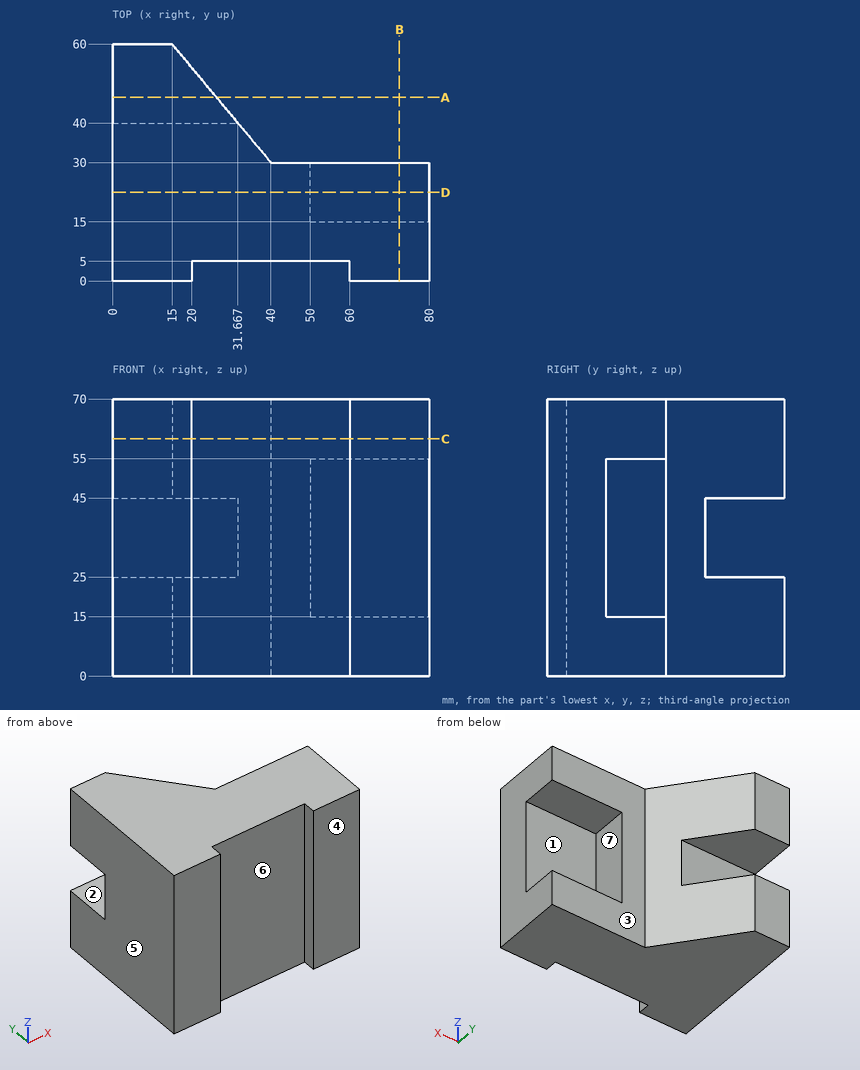
The drawing under review shows one solid part. Ordinate dimensions are in mm from its lowest x, y, z. A direction names the side the tool comes from. Give positions to 0.01 mm unless a question says otherwise; leave off trailing zeros. Loops run counter-clockwise (first coordinate to the right, second up) from the corner with the lowest first, then second, coordinate; pieces in that order, holes last. Notation, with made-up numbers: M 54,86 L 80,86 A22 ccw 80,108 Z; hole C 46,-32 d8. An arc over 180 degrees is marked long. One line per item, written item: value. Start each with the question number.
Q1. Add section C-C (z = 60). Give the boundary of the cut face in (x, y).
Q2. Draft analysis for pull direction X (two halves, no side actions). For the marked faces 4, 5, 6 and 7, state which applies: released by +X, released by -X, zero draft, split by the parting line, or undercut.
Q3. Machinability: for the marked faces 1, 2 and 3, which of the approach directions +Z, -Z, +X, -X, +Y, -Y give a long, thin tool a straight path to every point of the face, cutting with its end or side? Answer none if there is none.
Q4. For L1, parallel to Z at x = 62.5, y = 22; L2, parallel to Y at x = 24, z = 38; L3, parallel to Y at x = 53, z = 39.5, list the stretches that pass through material, from the lowest coordinate up.
Q5. Add section B-B (x = 72.5). Give the boundary of the cut face in (y, z), and give its area (3 significant figures).
Q6. Add section A-A (y = 46.5). Give the boundary of the cut face in (x, z), and give its area (3 significant figures).
Q7. Clearance check with flat-ended pins moving along their axes: pin 1 Ø12 at (x, y) = (60.5, 37.5) entering from +Z; pin 2 Ø20 at (x, z) = (48.5, 30.5) entering from -Y; pin 3 Ø12 at (x, z) = (69, 14.5) entering from +Y; pin 4 Ø1 at (y, z) = (42, 50) entering from +X. State where each tip first meets the part, or that it passes through.
Q8. Add section D-D (y = 22.5). Give the boundary of the cut face in (x, z).
Reply:
1. outline: M 0,0 L 20,0 L 20,5 L 60,5 L 60,0 L 80,0 L 80,30 L 40,30 L 15,60 L 0,60 Z
2. face 4: zero draft
2. face 5: released by -X
2. face 6: undercut
2. face 7: released by +X
3. face 1: +X, +Y
3. face 2: +X, -X, +Y
3. face 3: +Z, -Z, +X, +Y
4. L1: 0 to 15, 55 to 70
4. L2: 5 to 40
4. L3: 5 to 15
5. outline: M 0,0 L 30,0 L 30,15 L 15,15 L 15,55 L 30,55 L 30,70 L 0,70 Z
5. area: 1,500 mm²
6. outline: M 0,0 L 26.25,0 L 26.25,25 L 0,25 Z; M 0,45 L 26.25,45 L 26.25,70 L 0,70 Z
6. area: 1,310 mm²
7. pin 1: through
7. pin 2: y = 5
7. pin 3: y = 30
7. pin 4: x = 30.42
8. outline: M 0,0 L 80,0 L 80,15 L 50,15 L 50,55 L 80,55 L 80,70 L 0,70 Z
